Geometry check sheet. Reference: the model listing, model coordinates, mm. A direction names the side the tool comes from. Give positions to 0.01 mm unless a question says otherwise; leave off trailing zeros. Order: outer loops, then holes, each group sorted by start corner. A loop starts at its lowest first (then second) coordinate and runs counter-clockwise, first axis right, second up. Notation, with made-up numbers: M 62.25,73 L 93.25,73 A14 ccw 93.25,99 Z; hole C 76,25.5 d1. An arc over 180 degrees is marked long. Put each result on its own line as item: value. Start each with the question number.
Q1. Go/stop test with flat-tipped pins: pin 1 (8 mm diameter, centred on x = 14.5, z = -12, fed in from -Y); pin 2 (2 mm diameter, centred on x = 12.5, y = 6, fed in from +Z); pin 3 (1.6 mm diameter, centred on y = 6, z = -26.5, fed in from +X). Record where each tip stops, or that it passes through.
Q2. Section check D-D on z = 0. Record the cut outline in (x, y).
Q3. Mould release check, pull along X, two halves, no side actions. Record for faces 1 (the flat face through (2, 7, -26)), 2 (the flat face through (4, 0, 24)), 3 (the cylindrical face through (28.14, 3.7, 8.86)), 4 (the flat face through (-2, 7, -26)): +X half, -X half, draft (parallel to the pull), parting line (faces both ways), or undercut.
Q4. Section check A-A on x = 0. Record the cut outline in (y, z), then the cut area to 3 significant figures.
Q5. Access from +Z, -Z, +X, -X, +Y, -Y to the whole of each face (thin tool, end or side, straight path). Record for faces 5 (the cylindrical face through (-23.977, 0.493, 1.055)), 6 (the flat face through (0, 7.5, 0)), 7 (the cylindrical face through (-0.044, 6.514, -21.433)).
Q6. Material ranges on L1, parallel to Z at x = 0, y = 0.7; L2, parallel to Y at x = 5, z = 15.5; L3, parallel to X at y = 3, z = 21, recorded low to high.
Q7. Section check B-B on z = -13.5. Record the cut outline in (x, y), then the cut area to 3 significant figures.
Q8. Section check C-C on y = 3.5. Record the cut outline in (x, z), then the cut area to 3 significant figures.
Autodesk Fusion 360 part; units mm, degrees
sketch "草图1" plane through (0, 0, 0) normal (0, 1, 0) x (1, 0, 0)
  circle A0 centre (0, 0) radius 29.5
  line L0 (0, 0) -> (0, 29.5) construction
  dimension "d1" = 59
extrude "拉伸1" add sketch "草图1" along normal blind 7.5
sketch "草图2" plane through (0, 0, 0) normal (0, -1, 0) x (1, 0, 0)
  circle A0 centre (0, 0) radius 29.5
  circle A1 centre (0, 0) radius 24
  dimension "d5" = 48
  dimension "d6" = 48
extrude "拉伸2" cut sketch "草图2" against normal blind 1 contours A1
sketch "草图3" plane through (0, 7.5, 0) normal (0, 1, 0) x (-1, 0, 0)
  circle A0 centre (0, 0) radius 29.5
  line L0 (-2, -23.4321) -> (-2, -29.4321)
  line L1 (2, -23.4321) -> (2, -29.4321)
  line L2 (0, 0) -> (0, -21.4321) construction
  arc A1 (2, -23.4321) -> (-2, -23.4321) centre (0, -23.4321) ccw
  dimension "d9" = 6
  dimension "d10" = 2
  dimension "d11" = 6
  dimension "d12" = 2
  dimension "d13" = 2
extrude "拉伸3" cut sketch "草图3" against normal blind 2 contours A0 L0 L1 A1 picked at (0.2224, -25.4522)
Results found:
1. pin 1: stops at y = 1
1. pin 2: stops at z = 27.17
1. pin 3: stops at x = 14.48
2. outline: M -29.5,0 L -24,0 L -24,1 L 24,1 L 24,0 L 29.5,0 L 29.5,7.5 L -29.5,7.5 Z
3. face 1: undercut
3. face 2: draft
3. face 3: parting line
3. face 4: undercut
4. outline: M 0,-29.5 L 5.5,-29.5 L 5.5,-21.43 L 7.5,-21.43 L 7.5,29.5 L 0,29.5 L 0,24 L 1,24 L 1,-24 L 0,-24 Z
4. area: 378 mm^2
5. face 5: -Y
5. face 6: +Z, -Z, +X, -X, +Y
5. face 7: -Z, +Y
6. L1: z = -29.5 to -24, 24 to 29.5
6. L2: y = 1 to 7.5
6. L3: x = -20.72 to 20.72
7. outline: M -26.23,0 L -19.84,0 L -19.84,1 L 19.84,1 L 19.84,0 L 26.23,0 L 26.23,7.5 L -26.23,7.5 Z
7. area: 354 mm^2
8. outline: C 0,0 d59
8. area: 2,730 mm^2
